Could you check a few things on this model? Use its own coordinates, in mm. Give positions to 0.01 mm unless a question says otherwise; leave off trailing zeros. Write each loop counter-clockwise with the first axis right and the second up, starting at its lowest first coordinate (ties: lowest second). Pieces come first, ordered by that corner, then holes. Notation, with made-up numbers: M -27,74 L 25,74 A34 cw 25,112 Z; hole C 79.25,67 d5. An arc over 180 degrees is marked long. One line per item, written item: value.
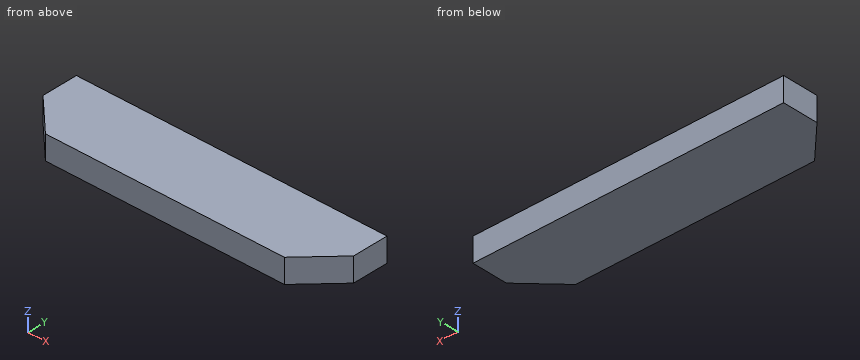
```python
from build123d import *

# Parameters (mm, degrees)
F0_W     = 150
F0_H     = 50
F1_DEPTH = 325
F3_DEPTH = 50.001


# Not quite as in the source:
# - a pattern or mirror of a feature is missing from the dataset's text; its kind, count and spacing are read off the source's solid


with BuildPart() as f1:
    # F0 (on Right) → F1 (new body, symmetric)
    with BuildSketch(Plane.YZ):
        Rectangle(F0_W, F0_H)
    extrude(amount=F1_DEPTH, both=True)

    # F2 (on face) → F3 (cut, through all)
    with BuildSketch(Plane.XY.offset(25)):
        Polygon((-250, -75), (-325, 0), (-325, -75), align=None)
    f3 = extrude(amount=-F3_DEPTH, mode=Mode.SUBTRACT)

    # F3_copies: F3 across plane
    add(f3.mirror(Plane(origin=(0, 0, 0), x_dir=(0, 0, 1), z_dir=(1, 0, 0))), mode=Mode.SUBTRACT)


solid = f1.part
```
1) If we section it at C-C, the plane y = -15: Write out the boundary of the cut face in (x, z), then the cut area to 3 significant figures.
Outcome:
outline: M -310,-25 L 310,-25 L 310,25 L -310,25 Z
area: 31,000 mm^2
2) If we section it at A-A, the plane z = 2: Write out the boundary of the cut face in (x, y), then the cut area to 3 significant figures.
Outcome:
outline: M -325,0 L -250,-75 L 250,-75 L 325,0 L 325,75 L -325,75 Z
area: 91,900 mm^2
3) I'm going to push flat-ended pins straight in: pin 1 (3 mm diameter, centred on y = -52, z = 14, fed in from -X); pin 2 (3 mm diameter, centred on y = -58.5, z = 5.5, fed in from -X); pin 3 (6 mm diameter, centred on y = -11.5, z = 10.5, fed in from +X). Where does each tip first touch, or does it pass through?
Outcome:
pin 1: stops at x = -274.5
pin 2: stops at x = -268
pin 3: stops at x = 316.5
4) If we section it at B-B, the plane y = -56.5: Write out the boundary of the cut face in (x, z), then the cut area to 4 significant figures.
Outcome:
outline: M -268.5,-25 L 268.5,-25 L 268.5,25 L -268.5,25 Z
area: 26,850 mm^2
5) Please list where these lines run through material, in increasing order: L1, parallel to Y at x = 256, z = 9; L2, parallel to X at y = -26, z = 10.5; L3, parallel to X at y = -9.5, z = 2.5. Write a range as from..to.
Outcome:
L1: y = -69..75
L2: x = -299..299
L3: x = -315.5..315.5
